Geometry check sheet. Reference: the model listing, model coordinates, mm. A direction names the side the tool comes from. Coordinates: 2 decimals unless noted, no trailing zeros. Loops run counter-clockwise (first coordinate to the right, second up) from the corner with the lowest first, then second, coordinate; pieces in that order, holes last.
from build123d import *

# Parameters (mm, degrees)
F1_DEPTH = 12.5
F3_DEPTH = 7.5
F4_R     = 2
F5_R     = 2
F8_D     = 60
F9_D     = 30
F10_R    = 5


with BuildPart() as f1:
    # F0 (on Front) → F1 (new body)
    with BuildSketch(Plane.XZ):
        with BuildLine():
            ThreePointArc((-44.228067, -25.55559), (-37.377684, -13.585336), (-35, 0))
            ThreePointArc((-35, 0), (-37.377684, 13.585336), (-44.228067, 25.55559))
            ThreePointArc((-44.228067, 25.55559), (-115, 0), (-44.228067, -25.55559))
        make_face()
        with BuildLine():
            ThreePointArc((-44.228067, 25.55559), (-37.377684, 13.585336), (-35, 0))
            ThreePointArc((-35, 0), (-37.377684, -13.585336), (-44.228067, -25.55559))
            Line((-44.228067, -25.55559), (59.939192, -13.159486))
            ThreePointArc((59.939192, -13.159486), (55, 0), (59.939192, 13.159486))
            Line((59.939192, 13.159486), (-44.228067, 25.55559))
        make_face()
        with BuildLine():
            ThreePointArc((95, 0), (82.027938, 18.724532), (59.939192, 13.159486))
            ThreePointArc((59.939192, 13.159486), (55, 0), (59.939192, -13.159486))
            ThreePointArc((59.939192, -13.159486), (82.027938, -18.724532), (95, 0))
        make_face()
    extrude(amount=F1_DEPTH)

    # F2 (on face) → F3 (cut)
    with BuildSketch(Plane.XZ.offset(12.5)):
        with BuildLine():
            Line((54.674672, 10.764806), (-37.926643, 21.78454))
            ThreePointArc((-37.926643, 21.78454), (-32, 0), (-37.926643, -21.78454))
            Line((-37.926643, -21.78454), (54.674672, -10.764806))
            ThreePointArc((54.674672, -10.764806), (52, 0), (54.674672, 10.764806))
        make_face()
    extrude(amount=-F3_DEPTH, mode=Mode.SUBTRACT)

    # F4
    f4_edges = [f1.edges().sort_by_distance(p)[0] for p in [
        (-37.926643, -8.75, -21.78454),
        (54.674672, -8.75, 10.764806),
        (54.674672, -8.75, -10.764806),
        (-37.926643, -8.75, 21.78454),
    ]]
    fillet(f4_edges, radius=F4_R)

    # F5
    f5_edges = [f1.edges().sort_by_distance(p)[0] for p in [
        (8.908671, -5, 16.211048),
    ]]
    fillet(f5_edges, radius=F5_R)

    # F6: F1 across plane


with BuildPart() as f1_1:
    add(f1.part)
    add(f1.part.mirror(Plane.XZ))

    # F8 (through all)
    with Locations(Plane.XZ.offset(12.5)):
        with Locations((-75, 0)):
            Hole(F8_D / 2)

    # F9 (through all)
    with Locations(Plane.XZ.offset(12.5)):
        with Locations((75, 0)):
            Hole(F9_D / 2)

    # F10
    f10_edges = [f1_1.edges().sort_by_distance(p)[0] for p in [
        (-44.228067, -6.25, 25.55559),
        (59.939192, -6.25, 13.159486),
        (-44.228067, -6.25, -25.55559),
        (59.939192, -6.25, -13.159486),
    ]]
    fillet(f10_edges, radius=F10_R)


solid = f1_1.part
(1) Scan lines: L1, parallel to X at y = 1.25, z = -12; L2, parallel to X at y = -10, z = 3.5; L3, parallel to Z at x = -75, y = -1.25. Record each from-to range of solid material in increasing order.
Findings:
L1: x = -113.16 to -102.5, -47.5 to 66, 84 to 91
L2: x = -114.85 to -104.8, -45.2 to -32.14, 52.27 to 60.41, 89.59 to 94.69
L3: z = -40 to -30, 30 to 40
(2) Access from +Z, -Z, +X, -X, +Y, -Y to the whole of each face (thin tool, end or side, straight path). Record for faces 1 (the flat face through (8.292, -0.175, 19.306)), 2 (the cylindrical face through (8.239, 5.601, 15.716)), 3 (the cylindrical face through (52, -10, 0)), 4 (the flat face through (6.895, -0.175, -19.472)), 5 (the flat face through (-34, -12.5, 3)).
Findings:
face 1: +Z, +Y, -Y
face 2: +Y
face 3: -Y
face 4: -Z, +Y, -Y
face 5: +Z, -Z, +X, -X, -Y
(3) Draft check along X on faces 6 (the cylindrical face through (-114.977, -0.175, 1.345)), 7 (the flat face through (-34, 12.5, 3)), 8 (the flat face through (9.51, -9.79, 16.14)). Enter one of: +X half, -X half, draft (parallel to the pull), parting line (faces both ways), or undercut.
Findings:
face 6: parting line
face 7: draft
face 8: undercut
(4) Sectioned sample at B-B on y = -1. Record the cut outline in (x, z), and give its area (3 significant figures).
Findings:
outline: (-45.42, -26.93) arc R5 cw to (-42.31, -25.33) - (57.5, -13.45) arc R5 cw to (61.47, -14.73) arc R20 ccw (long way) to (61.47, 14.73) arc R5 cw to (57.5, 13.45) - (-42.31, 25.33) arc R5 cw to (-45.42, 26.93) arc R40 ccw (long way) to start; hole circle Ø60 at (-75, 0); hole circle Ø30 at (75, 0)
area: 6,370 mm2
(5) Sectioned sample at C-C on z = -23.5. Record the cut outline in (x, y), and give its area (3 significant figures).
Findings:
outline: (-107.37, -12.5) - (-93.65, -12.5) - (-93.65, 12.5) - (-107.37, 12.5) - close; (-56.35, -12.5) - (-26.95, -12.5) - (-26.95, 12.5) - (-56.35, 12.5) - close
area: 1,080 mm2
(6) Sectioned sample at D-D on y = 9.5. Record the cut outline in (x, z).
Findings:
outline: (-45.42, -26.93) arc R5 cw to (-42.31, -25.33) - (57.5, -13.45) arc R5 cw to (61.47, -14.73) arc R20 ccw (long way) to (61.47, 14.73) arc R5 cw to (57.5, 13.45) - (-42.31, 25.33) arc R5 cw to (-45.42, 26.93) arc R40 ccw (long way) to start; hole circle Ø60 at (-75, 0); hole (-36.18, -18.49) arc R2 ccw to (-34.14, -21.33) - (51.95, -11.09) arc R2 ccw to (53.58, -8.37) arc R23 cw to (53.58, 8.37) arc R2 ccw to (51.95, 11.09) - (-34.14, 21.33) arc R2 ccw to (-36.18, 18.49) arc R43 cw to start; hole circle Ø30 at (75, 0)
(7) Sectioned sample at A-A on x = -75. Record the cut outline in (y, z).
Findings:
outline: (-12.5, -40) - (12.5, -40) - (12.5, -30) - (-12.5, -30) - close; (-12.5, 30) - (12.5, 30) - (12.5, 40) - (-12.5, 40) - close
(8) Gauge pin test, flat ends, axial feed: pin 1 Ø12 at (x, z) = (51, -23) entering from +Y; pin 2 Ø6 at (x, y) = (5, 10) entering from -Z; pin 3 Ø12 at (x, y) = (-53, 10) entering from -Z; pin 4 Ø1 at (y, z) = (9.5, -26.5) entering from -X. Record the tip position at first contact, or that the pin passes through.
Findings:
pin 1: passes through
pin 2: stops at z = -20.05
pin 3: stops at z = -36.66
pin 4: stops at x = -105.4
